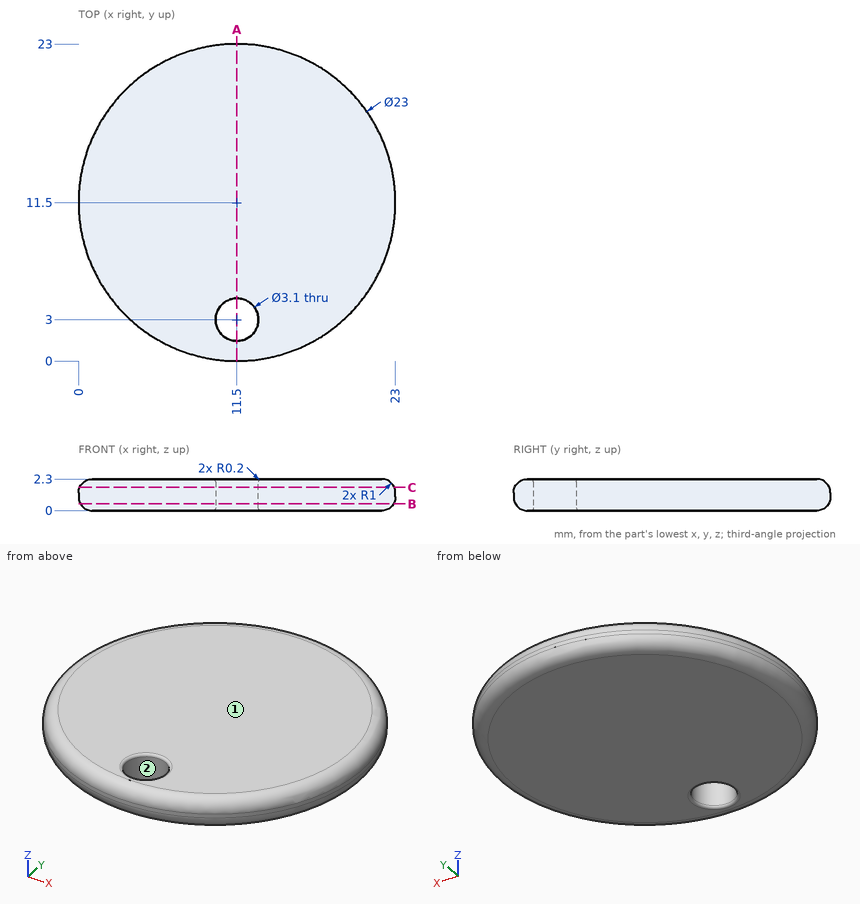
Here's the drawing with two shaded views (mm, measured from the low corner). I have some questions. Coordinates: 2 decimals unless noted, no trailing zeros. Write each loop counter-clockwise with the first axis right and the second up, starting at its lowest first coordinate (ties: lowest second). Pieces come first, ordered by that corner, then holes. Notation, with made-up numbers: M 31.5,66 L 36.5,66 A12 ccw 36.5,89 Z; hole C 22,-21 d2. An arc over 180 degrees is marked long. Use one line per item in the form item = value.
Q1. If we section it at B-B (z = 0.5): Write out the boundary of the cut face in (x, y).
Model answer:
outline = C 11.5,11.5 d22.73; hole C 11.5,3 d3.1
Q2. We'd pull the mould along X, two halves only. Please class the marked faces 1 and 2: +X half, -X half, draft (parallel to the pull), parting line (faces both ways), or undercut.
Model answer:
face_1 = draft
face_2 = undercut
Q3. I need wall thicknesses on line 1 along Y through (x, z) = (11.5, 1.3); line 2 along X through (y, z) = (12.25, 0.8); line 3 along Y through (x, z) = (16.75, 1.65). Which ranges of each line are inside material? Lowest first, please. Write a range as from..to.
Model answer:
line_1 = 0..1.45, 4.55..23
line_2 = 0.04..22.96
line_3 = 1.34..21.66
Q4. If we section it at A-A (x = 11.5): Write out the boundary of the cut face in (y, z), then the cut area to 3 significant figures.
Model answer:
outline = M 0,1 A1 ccw 1,0 L 1.25,0 A0.2 ccw 1.45,0.2 L 1.45,2.1 A0.2 ccw 1.25,2.3 L 1,2.3 A1 ccw 0,1.3 Z; M 4.55,0.2 A0.2 ccw 4.75,0 L 22,0 A1 ccw 23,1 L 23,1.3 A1 ccw 22,2.3 L 4.75,2.3 A0.2 ccw 4.55,2.1 Z
area = 44.9 mm^2
Q5. For P1, Ø1.9, axis at x = 11.5, y = 3, coming from the -Z side, with a flat end and sliding along its axis, tell me the tip position at first contact or that it passes through.
Model answer:
P1 = through
Q6. If we section it at C-C (z = 1.7): Write out the boundary of the cut face in (x, y).
Model answer:
outline = C 11.5,11.5 d22.83; hole C 11.5,3 d3.1
